Autodesk Inventor part; units mm, degrees
ref_plane "YZ Plane" through (0, 0, 0) normal (1, 0, 0) x (0, 1, 0)
ref_plane "XZ Plane" through (0, 0, 0) normal (0, 1, 0) x (-1, 0, 0)
ref_plane "XY Plane" through (0, 0, 0) normal (0, 0, 1) x (1, 0, 0)
sketch "Sketch1" plane through (0, 0, 0) normal (0, 1, 0) x (-1, 0, 0)
  line L0 (-16.95, -16.95) -> (16.95, -16.95)
  line L1 (16.95, -16.95) -> (16.95, 16.95)
  line L2 (16.95, 16.95) -> (-16.95, 16.95)
  line L3 (-16.95, 16.95) -> (-16.95, -16.95)
  line L4 (-16.95, -16.95) -> (16.95, 16.95) construction
  line L5 (16.95, -16.95) -> (-16.95, 16.95) construction
  line L6 (-15, -15) -> (15, -15)
  line L7 (15, -15) -> (15, 15)
  line L8 (15, 15) -> (-15, 15)
  line L9 (-15, 15) -> (-15, -15)
  line L10 (-15, -15) -> (15, 15) construction
  line L11 (15, -15) -> (-15, 15) construction
  point P0 (0, 0)
  dimension "d0" = 33.9
  dimension "d1" = 33.9
  dimension "d2" = 30
  dimension "d3" = 30
extrude "Extrusion1" add sketch "Sketch1" along normal blind 48
fillet "Fillet1" radius 2 4 edges at (16.95, 24, 16.95) (16.95, 24, -16.95) (-16.95, 24, -16.95) (-16.95, 24, 16.95)
properties part number "00_Laser_match_housing"
Build history of the part. All positions in model axes, mm. A direction names the side the tool comes from. Give positions to 0.01 mm unless a question says otherwise; leave off trailing zeros. Order: outer loops, then holes, each group sorted by start corner. A loop starts at its lowest first (then second) coordinate and runs counter-clockwise, first axis right, second up. Notation, with made-up numbers: M 89,16 L 105,16 A32 ccw 105,51 Z; hole C 23.5,-6 d9. An arc over 180 degrees is marked long. Return JSON: item names as keys, results as strings.
Q1. 3-axis set-ups, long thin cutter, end or side, ignore diameter. For faces 5 (the face through (-16.35, 24.34, -16.38)), 6 (the face through (0, 24, 15)): which of +Z, -Z, +X, -X, +Y, -Y reach the whole face in a straight line?
Answer list:
{"face 5": "-Z, -X, +Y, -Y", "face 6": "+Y, -Y"}
Q2. Band-saw the part on B-B (y = 8.5). Give the cut face in (x, z).
Answer list:
{"outline": "M -16.95,-14.95 A2 ccw -14.95,-16.95 L 14.95,-16.95 A2 ccw 16.95,-14.95 L 16.95,14.95 A2 ccw 14.95,16.95 L -14.95,16.95 A2 ccw -16.95,14.95 Z; hole M -15,-15 L 15,-15 L 15,15 L -15,15 Z"}
Q3. Band-saw the part on A-A (x = 0). Give the cut face in (y, z), then the cut area to 3 significant figures.
Answer list:
{"outline": "M 0,-16.95 L 48,-16.95 L 48,-15 L 0,-15 Z; M 0,15 L 48,15 L 48,16.95 L 0,16.95 Z", "area": "187 mm^2"}
Q4. Wall check: probe 1 along X at (y, z) = (11, 8). Give the ranges that are in metal, low to high. Write a range as from..to.
Answer list:
{"probe 1": "x = -16.95..-15, 15..16.95"}
Q5. Two-plate mould, pull along Z, no slides. Class faces 1 (the face through (-15, 24, 0)), 2 (the face through (2.59, 48, 15.15)), 3 (the face through (15, 24, 0)), 4 (the face through (0, 24, -16.95)): pulls with the +Z half, pulls with the -Z half, needs draft (parallel to the pull), parting line crosses it, or undercut.
Answer list:
{"face 1": "undercut", "face 2": "needs draft", "face 3": "undercut", "face 4": "pulls with the -Z half"}
Q6. Band-saw the part on C-C (z = 14). Give the cut face in (x, y), then the cut area to 3 significant figures.
Answer list:
{"outline": "M -16.95,0 L -15,0 L -15,48 L -16.95,48 Z; M 15,0 L 16.95,0 L 16.95,48 L 15,48 Z", "area": "187 mm^2"}
